Input: part model. Units: mm. Frame: model coordinates. Face numbers are marked on the shaded views. Coordinates: 2 decimals unless noted, no trailing zeros. Loops run counter-clockwise (first coordinate to the right, second up) from the corner with the lowest first, then second, coordinate; pieces in that order, holes last. Notation, with made-up numbers: (3.5, 54) -> (14.5, 54) arc R34 cw to (14.5, 90) -> close; hole circle Ø1 at (17, 34.5). An arc over 180 degrees is marked (long way). Put each result on its own line as item: value. Start each with the question number.
1) Cut plane D-D (y = 14). Return the cut outline in (x, z).
2) Contact query for flat-ended pins moving along their axis: P1, Ø6, axis at x = 2, y = 4.5, coming from the -Z side; P2, Ø1, axis at x = -1.5, y = -25, coming from the +Z side. Output: stop coordinate, or through.
3) Material intervals for L1, parallel to Z at x = 6.25, y = 1.5; L2, parallel to Y at x = -0.75, z = 0; L3, parallel to Y at x = 6, z = -39, sorted ascending.
4) Cut plane C-C (x = 4.75). Return the cut outline in (y, z) (1 decimal), plus the area to 3 significant figures.
5) Cut plane A-A (y = 0). Return the cut outline in (x, z).
6) Pull-direction query (Y, two-part tool) for the marked faces 1 and 2; classes: pulls with the +Y half, pulls with the -Y half, needs draft (parallel to the pull), parting line crosses it, or undercut.
7) Cut plane B-B (z = 0). Return the cut outline in (x, y), plus the area to 3 significant figures.
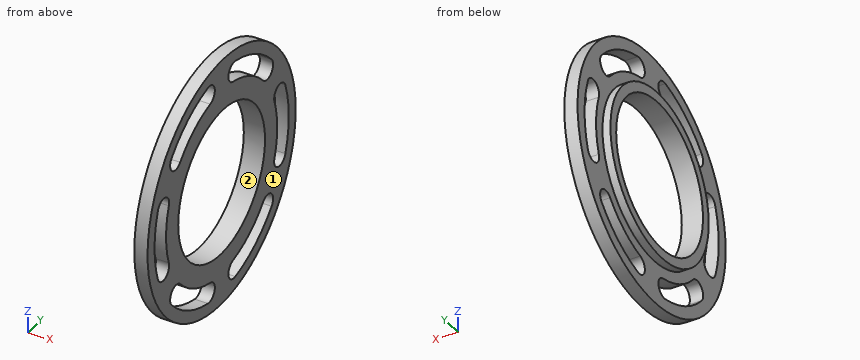
from build123d import *

# Parameters (mm, degrees)
CUT_EXTRUDE1_DEPTH = 87.981371925
CIRPATTERN1_COUNT  = 6


with BuildPart() as part:
    # Sketch2 → Revolve1 (revolve)
    with BuildSketch(Plane.XY, mode=Mode.PRIVATE) as revolve1_sk:
        Polygon((0, 35.941), (6.35, 35.941), (6.35, 61.341), (0, 61.341), (0, 40.7035), (-3.81, 40.7035), (-3.81, 35.941), align=None)
    revolve(revolve1_sk.sketch.rotate(Axis((88.99, 0, 0), (-1, 0, 0)), 90), axis=Axis((88.99, 0, 0), (-1, 0, 0)))

    # Sketch3 → Cut-Extrude1 (cut, through all)
    with BuildSketch(Plane(origin=(0, 0, 0), x_dir=(0, 0, -1), z_dir=(1, 0, 0))):
        with BuildLine():
            ThreePointArc((17.36328125, 52.779805518), (0, 55.5625), (-17.36328125, 52.779805518))
            ThreePointArc((-17.36328125, 52.779805518), (-20.39898333, 46.767540938), (-14.38671875, 43.731838858))
            ThreePointArc((-14.38671875, 43.731838858), (0, 46.0375), (14.38671875, 43.731838858))
            ThreePointArc((14.38671875, 43.731838858), (20.39898333, 46.767540938), (17.36328125, 52.779805518))
        make_face()
    cut_extrude1 = extrude(amount=CUT_EXTRUDE1_DEPTH, mode=Mode.SUBTRACT)

    # CirPattern1: Cut-Extrude1 ×6 about axis
    cirpattern1_axis = Axis((0, 0, 0), (1, 0, 0))
    for i in range(1, CIRPATTERN1_COUNT):
        add(cut_extrude1.rotate(cirpattern1_axis, i * 360 / CIRPATTERN1_COUNT), mode=Mode.SUBTRACT)


solid = part.part
Results found:
1. outline: (-3.81, -38.22) -> (0, -38.22) -> (0, -43.86) -> (6.35, -43.86) -> (6.35, -33.1) -> (-3.81, -33.1) -> close; (-3.81, 33.1) -> (6.35, 33.1) -> (6.35, 43.86) -> (0, 43.86) -> (0, 38.22) -> (-3.81, 38.22) -> close; (0, -59.72) -> (6.35, -59.72) -> (6.35, -53.77) -> (0, -53.77) -> close; (0, 53.77) -> (6.35, 53.77) -> (6.35, 59.72) -> (0, 59.72) -> close
2. P1: stops at z = -61.32
2. P2: stops at z = 32.5
3. L1: z = -61.32 to -35.91, 35.91 to 61.32
3. L2: y = -40.7 to -35.94, 35.94 to 40.7
3. L3: y = -47.35 to -39.58, -24.46 to 24.46, 39.58 to 47.35
4. outline: circle Ø122.7 at (0, 0); hole (-52.8, -17.4) arc R4.8 ccw to (-43.7, -14.4) arc R46 cw to (-43.7, 14.4) arc R4.8 ccw to (-52.8, 17.4) arc R55.6 ccw to start; hole (-41.4, -37) arc R55.6 ccw to (-11.4, -54.4) arc R4.8 ccw to (-9.4, -45.1) arc R46 cw to (-34.3, -30.7) arc R4.8 ccw to start; hole (-41.4, 37) arc R4.8 ccw to (-34.3, 30.7) arc R46 cw to (-9.4, 45.1) arc R4.8 ccw to (-11.4, 54.4) arc R55.6 ccw to start; hole circle Ø71.9 at (0, 0); hole (9.4, -45.1) arc R4.8 ccw to (11.4, -54.4) arc R55.6 ccw to (41.4, -37) arc R4.8 ccw to (34.3, -30.7) arc R46 cw to start; hole (9.4, 45.1) arc R46 cw to (34.3, 30.7) arc R4.8 ccw to (41.4, 37) arc R55.6 ccw to (11.4, 54.4) arc R4.8 ccw to start; hole (43.7, -14.4) arc R4.8 ccw to (52.8, -17.4) arc R55.6 ccw to (52.8, 17.4) arc R4.8 ccw to (43.7, 14.4) arc R46 cw to start
4. area: 5,490 mm2
5. outline: (-3.81, -40.7) -> (0, -40.7) -> (0, -61.34) -> (6.35, -61.34) -> (6.35, -35.94) -> (-3.81, -35.94) -> close; (-3.81, 35.94) -> (6.35, 35.94) -> (6.35, 61.34) -> (0, 61.34) -> (0, 40.7) -> (-3.81, 40.7) -> close
6. face 1: needs draft
6. face 2: undercut
7. outline: (-3.81, -40.7) -> (0, -40.7) -> (0, -46.04) -> (6.35, -46.04) -> (6.35, -35.94) -> (-3.81, -35.94) -> close; (-3.81, 35.94) -> (6.35, 35.94) -> (6.35, 46.04) -> (0, 46.04) -> (0, 40.7) -> (-3.81, 40.7) -> close; (0, -61.34) -> (6.35, -61.34) -> (6.35, -55.56) -> (0, -55.56) -> close; (0, 55.56) -> (6.35, 55.56) -> (6.35, 61.34) -> (0, 61.34) -> close
7. area: 238 mm2
